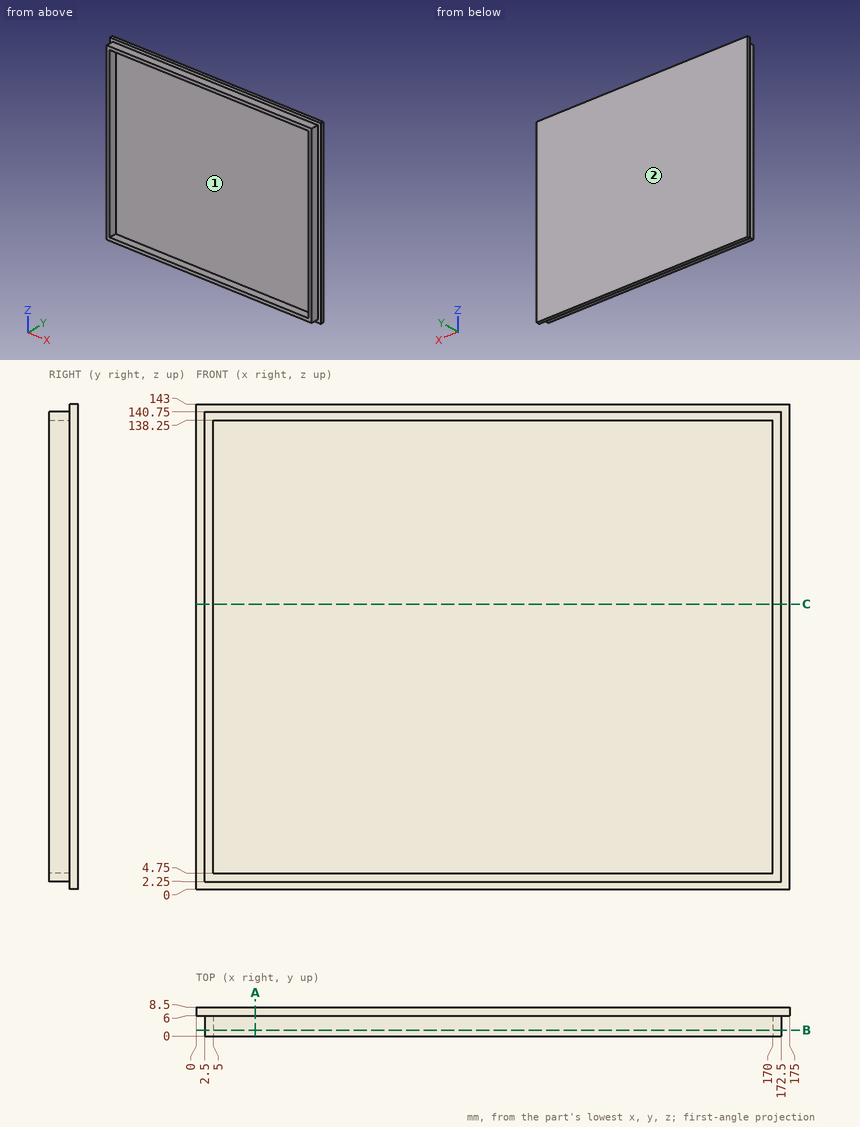
Study the drawing (mm; zero at the part's minimum x, y, z) and answer. Round coordinates to 2 decimals unless told otherwise and drop trailing zeros. Loops run counter-clockwise (first coordinate to the right, second up) from the corner with the lowest first, then second, coordinate; pieces in that order, holes last. Notation, with made-up numbers: (69.25, 34.5) - (122.25, 34.5) arc R31 cw to (122.25, 61.5) - close; hole circle Ø8 at (-19.5, 32). An arc over 180 degrees is marked (long way). Use one line per item in the form item = value. Start each with the question number.
1. The part is cut by section B-B on y = 1.75. Determine the outline of the cut face in (x, z), then the cut area to 3 significant figures.
2. Given pin 1 Ø5 at (y, z) = (2, 70.5) entering from -X; pin 2 Ø1.8 at (x, y) = (75.5, 2) entering from +Z; pin 3 Ø1.8 at (y, z) = (4, 48.5) entering from +X, each flat-ended and moving along its own axis, determine where each tip first touches the part or whether it passes through.
3. Consider line 1 (X direction, y = 4, z = 75.5); line 2 (Z direction, x = 129, y = 4.25); line 3 (Y direction, x = 104, z = 9). Determine where each line is inside the solid, lowest interval first. Write a range as [from, to].
4. For a pull along Z with two mould halves and no side action, classify the marked faces 1 and 2 as pulls with the +Z half, pulls with the -Z half, needs draft (parallel to the pull), parting line crosses it, or undercut.
5. The part is cut by section C-C on z = 84. Determine the outline of the cut face in (x, y).
6. The part is cut by section A-A on x = 17.5. Determine the outline of the cut face in (y, z), then the cut area to 4 significant figures.
Geometry check:
q1.outline = (2.5, 2.25) - (172.5, 2.25) - (172.5, 140.75) - (2.5, 140.75) - close; hole (5, 4.75) - (170, 4.75) - (170, 138.25) - (5, 138.25) - close
q1.area = 1,520 mm^2
q2.pin_1 = 2.5
q2.pin_2 = 140.75
q2.pin_3 = 172.5
q3.line_1 = [2.5, 5], [170, 172.5]
q3.line_2 = [2.25, 4.75], [138.25, 140.75]
q3.line_3 = [6, 8.5]
q4.face_1 = undercut
q4.face_2 = needs draft
q5.outline = (0, 6) - (2.5, 6) - (2.5, 0) - (5, 0) - (5, 6) - (170, 6) - (170, 0) - (172.5, 0) - (172.5, 6) - (175, 6) - (175, 8.5) - (0, 8.5) - close
q6.outline = (0, 2.25) - (6, 2.25) - (6, 0) - (8.5, 0) - (8.5, 143) - (6, 143) - (6, 140.75) - (0, 140.75) - (0, 138.25) - (6, 138.25) - (6, 4.75) - (0, 4.75) - close
q6.area = 387.5 mm^2
